Source: CAD feature listing. Evaluate the final solid. Frame: model axes, mm. A direction names the side the tool comes from. Give positions to 0.01 mm unless a question says otherwise; leave off trailing zeros. Write each loop counter-clockwise with the first axis right and the second up, starting at its lowest first coordinate (ties: lowest second). Pieces come first, ordered by that corner, then holes. Notation, with made-up numbers: (81, 44) -> (98, 44) arc R21 ccw to (98, 48) -> close; hole circle Ø4 at (-25.75, 62.25). An arc over 180 degrees is marked (long way). Answer as a JSON object with one key per item and string values. Group by question number.
Item 1: Section query D-D on x = 0. Return the cut outline in (y, z), plus the area to 3 significant figures.
Item 2: Access query for faces 4 (the face through (5, 17, 2)), 5 (the face through (14.141, 6.797, -0.493)), 6 (the face through (5, -17, 2)), 7 (the face through (-1, -16.5, 2)). Directions: +Z, -Z, +X, -X, +Y, -Y. A direction counts if a zero-diameter tool reaches every point of the face in a straight line with its end or side. Return the directions, or none.
Item 3: Ray query, probe 1 along Y at (x, z) = (-25, -0.6); probe 2 along Z at (x, y) = (2, -13); probe 3 along Z at (x, y) = (0, 16.95). Return the intervals inside material, ascending. Write a range as from..to.
Item 4: Section query C-C on x = -15. Return the cut outline in (y, z), plus the area to 3 significant figures.
Item 5: First-contact query: pin 1 Ø0.8 at (y, z) = (-16.5, -0.5) entering from +X; pin 2 Ø0.5 at (y, z) = (17, -0.5) entering from +X; pin 3 Ø1.8 at (y, z) = (16, 2.5) entering from -X. Flat tips, straight axial feed; report the tip coordinate or a pass-through.
Item 6: Pull-direction query (X, two-part tool) for faces 1 (the face through (1, 17.5, 2)), 2 (the face through (30.14, -8.9, -0.49)), 3 (the face through (-5, 17, 2)); classes: pulls with the +X half, pulls with the -X half, needs draft (parallel to the pull), parting line crosses it, or undercut.
Item 7: Section query A-A on y = 12.75. Return the cut outline in (x, z).
Item 8: Section query B-B on z = 9. Return the cut outline in (x, y), plus the area to 3 significant figures.
from build123d import *

# Parameters (mm, degrees)
SKETCH1_R                     = 1.5
BASE_FLANGE1_DEPTH            = 1
EDGE_FLANGE1_STRIP_W          = 5.4732
EDGE_FLANGE1_STRIP_H          = 1
EDGE_FLANGE1_STRIP_CUT_DEPTH  = 10
EDGE_FLANGE1_RELIEF_W         = 5.9732
EDGE_FLANGE1_RELIEF_H         = 0.5
EDGE_FLANGE1_RELIEF_CUT_DEPTH = 1
EDGE_FLANGE1_DEPTH            = 10
EDGE_FLANGE1_PROFILE_R        = 2.75
EDGE_FLANGE1_FLAT_DEPTH       = 1
EDGE_FLANGE2_STRIP_W          = 5.4732
EDGE_FLANGE2_STRIP_H          = 1
EDGE_FLANGE2_STRIP_CUT_DEPTH  = 10
EDGE_FLANGE2_RELIEF_W         = 5.9732
EDGE_FLANGE2_RELIEF_H         = 0.5
EDGE_FLANGE2_RELIEF_CUT_DEPTH = 1
EDGE_FLANGE2_DEPTH            = 10
EDGE_FLANGE2_PROFILE_R        = 2.75
EDGE_FLANGE2_FLAT_DEPTH       = 1


# Sheet-metal steps are written as plain solids
with BuildPart() as part:
    # Sketch1 → Base-Flange1 (new body)
    with BuildSketch(Plane.XY):
        with BuildLine():
            Line((-28, 8), (-17, 8))
            ThreePointArc((-17, 8), (-14.171572875, 6.828427125), (-13, 4))
            Line((-13, 4), (-13, -4))
            ThreePointArc((-13, -4), (-14.171572875, -6.828427125), (-17, -8))
            Line((-17, -8), (-28, -8))
            ThreePointArc((-28, -8), (-30.121320344, -8.878679656), (-31, -11))
            Line((-31, -11), (-31, -14.5))
            ThreePointArc((-31, -14.5), (-30.121320344, -16.621320344), (-28, -17.5))
            Line((-28, -17.5), (28, -17.5))
            ThreePointArc((28, -17.5), (30.121320344, -16.621320344), (31, -14.5))
            Line((31, -14.5), (31, -11))
            ThreePointArc((31, -11), (30.121320344, -8.878679656), (28, -8))
            Line((28, -8), (17, -8))
            ThreePointArc((17, -8), (14.171572875, -6.828427125), (13, -4))
            Line((13, -4), (13, 4))
            ThreePointArc((13, 4), (14.171572875, 6.828427125), (17, 8))
            Line((17, 8), (28, 8))
            ThreePointArc((28, 8), (30.121320344, 8.878679656), (31, 11))
            Line((31, 11), (31, 14.5))
            ThreePointArc((31, 14.5), (30.121320344, 16.621320344), (28, 17.5))
            Line((28, 17.5), (-28, 17.5))
            ThreePointArc((-28, 17.5), (-30.121320344, 16.621320344), (-31, 14.5))
            Line((-31, 14.5), (-31, 11))
            ThreePointArc((-31, 11), (-30.121320344, 8.878679656), (-28, 8))
        make_face()
        with Locations((-25, 12.75)):
            Circle(SKETCH1_R, mode=Mode.SUBTRACT)
        with Locations((25, 12.75)):
            Circle(SKETCH1_R, mode=Mode.SUBTRACT)
        with Locations((25, -12.75)):
            Circle(SKETCH1_R, mode=Mode.SUBTRACT)
        with Locations((-25, -12.75)):
            Circle(SKETCH1_R, mode=Mode.SUBTRACT)
    extrude(amount=-BASE_FLANGE1_DEPTH)

    # Edge-Flange1 strip (across the edge) → Edge-Flange1 strip cut (cut)
    with BuildSketch(Plane(origin=(5, 17.5, 0), x_dir=(0, -1, 0), z_dir=(-1, 0, 0))):
        with Locations((-1, -0.5)):
            Rectangle(EDGE_FLANGE1_STRIP_W, EDGE_FLANGE1_STRIP_H)
    extrude(amount=EDGE_FLANGE1_STRIP_CUT_DEPTH, mode=Mode.SUBTRACT)

    # Edge-Flange1 relief (on the sheet) → Edge-Flange1 relief cut (cut)
    with BuildSketch(Plane(origin=(5, 15.7634, 0), x_dir=(0, -1, 0), z_dir=(0, 0, 1))):
        with Locations((-2.4866, 0.25)):
            Rectangle(EDGE_FLANGE1_RELIEF_W, EDGE_FLANGE1_RELIEF_H)
        with Locations((-2.4866, -10.25)):
            Rectangle(EDGE_FLANGE1_RELIEF_W, EDGE_FLANGE1_RELIEF_H)
    extrude(amount=-EDGE_FLANGE1_RELIEF_CUT_DEPTH, mode=Mode.SUBTRACT)

    # Edge-Flange1 bend section (across the edge) → Edge-Flange1 (add)
    with BuildSketch(Plane(origin=(5, 17.5, 0), x_dir=(0, -1, 0), z_dir=(-1, 0, 0))):
        with BuildLine():
            Line((0, 0.7366), (1, 0.7366))
            ThreePointArc((1, 0.7366), (1.215745145, 0.215745145), (1.7366, 0))
            Line((1.7366, 0), (1.7366, -1))
            ThreePointArc((1.7366, -1), (0.508638364, -0.491361636), (0, 0.7366))
        make_face()
    extrude(amount=EDGE_FLANGE1_DEPTH)

    # Edge-Flange1 profile (on flange) → Edge-Flange1 flat (add)
    with BuildSketch(Plane(origin=(0, 17.5, 0), x_dir=(-1, 0, 0), z_dir=(0, 1, 0))):
        with BuildLine():
            Line((-5, 5), (-5, 0.7366))
            Line((-5, 0.7366), (5, 0.7366))
            Line((5, 0.7366), (5, 5))
            ThreePointArc((5, 5), (0, 10), (-5, 5))
        make_face()
        with Locations((0, 5)):
            Circle(EDGE_FLANGE1_PROFILE_R, mode=Mode.SUBTRACT)
    extrude(amount=-EDGE_FLANGE1_FLAT_DEPTH)

    # Edge-Flange2 strip (across the edge) → Edge-Flange2 strip cut (cut)
    with BuildSketch(Plane(origin=(-5, -17.5, 0), x_dir=(0, 1, 0), z_dir=(1, 0, 0))):
        with Locations((-1, -0.5)):
            Rectangle(EDGE_FLANGE2_STRIP_W, EDGE_FLANGE2_STRIP_H)
    extrude(amount=EDGE_FLANGE2_STRIP_CUT_DEPTH, mode=Mode.SUBTRACT)

    # Edge-Flange2 relief (on the sheet) → Edge-Flange2 relief cut (cut)
    with BuildSketch(Plane(origin=(-5, -15.7634, 0), x_dir=(0, 1, 0), z_dir=(0, 0, 1))):
        with Locations((-2.4866, 0.25)):
            Rectangle(EDGE_FLANGE2_RELIEF_W, EDGE_FLANGE2_RELIEF_H)
        with Locations((-2.4866, -10.25)):
            Rectangle(EDGE_FLANGE2_RELIEF_W, EDGE_FLANGE2_RELIEF_H)
    extrude(amount=-EDGE_FLANGE2_RELIEF_CUT_DEPTH, mode=Mode.SUBTRACT)

    # Edge-Flange2 bend section (across the edge) → Edge-Flange2 (add)
    with BuildSketch(Plane(origin=(-5, -17.5, 0), x_dir=(0, 1, 0), z_dir=(1, 0, 0))):
        with BuildLine():
            Line((0, 0.7366), (1, 0.7366))
            ThreePointArc((1, 0.7366), (1.215745145, 0.215745145), (1.7366, 0))
            Line((1.7366, 0), (1.7366, -1))
            ThreePointArc((1.7366, -1), (0.508638364, -0.491361636), (0, 0.7366))
        make_face()
    extrude(amount=EDGE_FLANGE2_DEPTH)

    # Edge-Flange2 profile (on flange) → Edge-Flange2 flat (add)
    with BuildSketch(Plane.XZ.offset(17.5)):
        with BuildLine():
            ThreePointArc((5, 5), (0, 10), (-5, 5))
            Line((-5, 5), (-5, 0.7366))
            Line((-5, 0.7366), (5, 0.7366))
            Line((5, 0.7366), (5, 5))
        make_face()
        with Locations((0, 5)):
            Circle(EDGE_FLANGE2_PROFILE_R, mode=Mode.SUBTRACT)
    extrude(amount=-EDGE_FLANGE2_FLAT_DEPTH)


solid = part.part
Worked answers:
{
 "1": {"outline": "(-17.5, 0.74) arc R1.74 ccw to (-15.76, -1) -> (15.76, -1) arc R1.74 ccw to (17.5, 0.74) -> (17.5, 2.25) -> (16.5, 2.25) -> (16.5, 0.74) arc R0.74 cw to (15.76, 0) -> (-15.76, 0) arc R0.74 cw to (-16.5, 0.74) -> (-16.5, 2.25) -> (-17.5, 2.25) -> close; (-17.5, 7.75) -> (-16.5, 7.75) -> (-16.5, 10) -> (-17.5, 10) -> close; (16.5, 7.75) -> (17.5, 7.75) -> (17.5, 10) -> (16.5, 10) -> close", "area": "42.9 mm^2"},
 "2": {"face 4": "+Z, -Z, +Y", "face 5": "+Z, -Z, +X", "face 6": "+Z, -Z, -Y", "face 7": "+Z, +X, -X"},
 "3": {"probe 1": "-17.5..-14.25, -11.25..-8, 8..11.25, 14.25..17.5", "probe 2": "-1..0", "probe 3": "-0.53..2.25, 7.75..10"},
 "4": {"outline": "(-17.5, -1) -> (-7.46, -1) -> (-7.46, 0) -> (-17.5, 0) -> close; (7.46, -1) -> (17.5, -1) -> (17.5, 0) -> (7.46, 0) -> close", "area": "20.1 mm^2"},
 "5": {"pin 1": "x = 30.54", "pin 2": "x = 29.98", "pin 3": "x = -5"},
 "6": {"face 1": "needs draft", "face 2": "pulls with the +X half", "face 3": "undercut"},
 "7": {"outline": "(-31, -1) -> (-26.5, -1) -> (-26.5, 0) -> (-31, 0) -> close; (-23.5, -1) -> (23.5, -1) -> (23.5, 0) -> (-23.5, 0) -> close; (26.5, -1) -> (31, -1) -> (31, 0) -> (26.5, 0) -> close"},
 "8": {"outline": "(-3, -17.5) -> (3, -17.5) -> (3, -16.5) -> (-3, -16.5) -> close; (-3, 16.5) -> (3, 16.5) -> (3, 17.5) -> (-3, 17.5) -> close", "area": "12.0 mm^2"}
}
